For this review, take the finished solid that the model builds, in its own axes (mm). A direction names the side the tool comes from. Round coordinates to 2 decimals unless told otherwise and drop trailing zeros. Order: outer loops, then holes, each group sorted by start corner. A loop starts at its lowest first (then second) coordinate and runs counter-clockwise, first axis right, second up. Notation, with made-up numbers: (45, 49.5) - (53, 49.5) arc R14 ccw to (53, 73.5) - close; hole circle Ø9 at (29, 42). An arc over 180 degrees is marked (long way). One line per item, written item: value.
Autodesk Inventor part; units mm, degrees
ref_plane "YZ Plane" through (0, 0, 0) normal (1, 0, 0) x (0, 1, 0)
ref_plane "XZ Plane" through (0, 0, 0) normal (0, 1, 0) x (-1, 0, 0)
ref_plane "XY Plane" through (0, 0, 0) normal (0, 0, 1) x (1, 0, 0)
sketch "Эскиз1" plane through (0, 0, 0) normal (0, 0, 1) x (1, 0, 0)
  line L0 (1380.315, -1246.7097) -> (1380.315, -1245.7097)
  line L1 (1390.315, -1235.7097) -> (1440.315, -1235.7097)
  line L2 (1450.315, -1245.7097) -> (1450.315, -1246.7097)
  arc A0 (1390.315, -1235.7097) -> (1380.315, -1245.7097) centre (1390.315, -1245.7097) ccw
  arc A1 (1450.315, -1245.7097) -> (1440.315, -1235.7097) centre (1440.315, -1245.7097) ccw
  line L3 (1380.315, -1246.7097) -> (1380.315, -1247.7097)
  line L4 (1372.315, -1255.7097) -> (1357.315, -1255.7097)
  line L5 (1473.3109, -1255.7097) -> (1458.315, -1255.7097)
  line L6 (1450.315, -1247.7097) -> (1450.315, -1246.7097)
  arc A2 (1372.315, -1255.7097) -> (1380.315, -1247.7097) centre (1372.315, -1247.7097) ccw
  arc A3 (1450.315, -1247.7097) -> (1458.315, -1255.7097) centre (1458.315, -1247.7097) ccw
  circle A4 centre (1415.315, -1239.7097) radius 2
  line L7 (1357.315, -1255.7097) -> (1356.315, -1255.7097)
  arc A5 (1356.315, -1255.7097) -> (1354.315, -1257.7097) centre (1356.315, -1257.7097) ccw
  line L8 (1473.3109, -1255.7097) -> (1474.3062, -1255.7097)
  arc A6 (1476.3062, -1257.7097) -> (1474.3062, -1255.7097) centre (1474.3062, -1257.7097) ccw
  circle A7 centre (1427.315, -1239.7097) radius 2
  arc A8 (1366.3109, -1262.2097) -> (1366.3109, -1266.2097) centre (1366.3109, -1264.2097) ccw
  arc A9 (1464.3109, -1266.2097) -> (1464.3109, -1262.2097) centre (1464.3109, -1264.2097) ccw
  line L9 (1366.3109, -1262.2097) -> (1464.3109, -1262.2097)
  line L10 (1464.3109, -1266.2097) -> (1366.3109, -1266.2097)
  line L11 (1366.315, -1269.7097) -> (1464.3062, -1269.7097)
  line L12 (1476.3062, -1257.7097) -> (1476.3062, -1257.7097)
  line L13 (1354.315, -1257.7097) -> (1354.315, -1257.7097)
  arc A10 (1354.315, -1257.7097) -> (1366.315, -1269.7097) centre (1366.315, -1257.7097) ccw
  arc A11 (1464.3062, -1269.7097) -> (1476.3062, -1257.7097) centre (1464.3062, -1257.7097) ccw
  circle A12 centre (1403.315, -1239.7097) radius 2
  point P0 (0, 0)
  point P1 (1450.315, -1235.7097)
  point P2 (1380.315, -1255.7097)
  point P3 (1354.315, -1255.7097)
  point P4 (1476.3109, -1270.2097)
extrude "Выдавливание3" add sketch "Эскиз1" along normal blind 2
properties part number "NEW Бампер"
Item 1: Take a section at C-C (z = 1.65). Write out the cut boundary in (x, y) (3 decimals), plus the area to 3 significant figures.
Returned:
outline: (1354.315, -1257.71) arc R12 ccw to (1366.315, -1269.71) - (1464.306, -1269.71) arc R12 ccw to (1476.306, -1257.71) arc R2 ccw to (1474.306, -1255.71) - (1458.315, -1255.71) arc R8 cw to (1450.315, -1247.71) - (1450.315, -1245.71) arc R10 ccw to (1440.315, -1235.71) - (1390.315, -1235.71) arc R10 ccw to (1380.315, -1245.71) - (1380.315, -1247.71) arc R8 cw to (1372.315, -1255.71) - (1356.315, -1255.71) arc R2 ccw to start; hole (1366.311, -1266.21) - (1464.311, -1266.21) arc R2 ccw to (1464.311, -1262.21) - (1366.311, -1262.21) arc R2 ccw to start; hole circle Ø4 at (1403.315, -1239.71); hole circle Ø4 at (1415.315, -1239.71); hole circle Ø4 at (1427.315, -1239.71)
area: 2,590 mm^2
Item 2: Wall thickness on line 1 (Y direction, x = 1418.5, z = 1.9); line 2 (Y direction, x = 1402.5, z = 0.5); line 3 (X direction, y = -1265, z = 0.2): over which ranges is each line inside the solid? List them lowest first.
Returned:
line 1: -1269.71 to -1266.21, -1262.21 to -1235.71
line 2: -1269.71 to -1266.21, -1262.21 to -1241.54, -1237.88 to -1235.71
line 3: 1356.78 to 1364.47, 1466.15 to 1473.84
Item 3: For P1, Ø0.6, axis at y = -1246.5, z = 1.5, coming from the +X side (3 decimals); P2, Ø0.6, axis at y = -1246.5, z = 1, coming from the -X side (3 decimals); P3, Ø1, axis at x = 1362.5, z = 0.5, coming from the +Y side, all flat-tipped, find the tip position at first contact; note any pin that passes through.
Returned:
P1: x = 1450.315
P2: x = 1380.315
P3: y = -1255.71
Item 4: Machinability: for faces 4 (the flat face through (1416, -1266.21, 1)), 5 (the flat face through (1450.315, -1247, 1)), 6 (the cylindrical face through (1357.924, -1266.288, 0.986)), 7 (the flat face through (1364, -1255.71, 1)), which of the approach directions +Z, -Z, +X, -X, +Y, -Y give a long, thin tool a straight path to every point of the face, cutting with its end or side? Answer none if there is none.
Returned:
face 4: +Z, -Z
face 5: +Z, -Z, +X, +Y
face 6: +Z, -Z, -X, -Y
face 7: +Z, -Z, -X, +Y
Item 5: The part is to be moulded in two halves that separate along Y. For faces 1 (the cylindrical face through (1452.72, -1253.43, 0.99)), 2 (the flat face through (1415, -1262.21, 1)), 3 (the flat face through (1414, -1252, 0)), say which applies: +Y half, -Y half, draft (parallel to the pull), parting line (faces both ways), or undercut.
Returned:
face 1: +Y half
face 2: undercut
face 3: draft
Item 6: Take a section at B-B (y = -1264). Write out the cut boundary in (x, z).
Returned:
outline: (1356.1, 0) - (1364.32, 0) - (1364.32, 2) - (1356.1, 2) - close; (1466.3, 0) - (1474.53, 0) - (1474.53, 2) - (1466.3, 2) - close
Item 7: Take a section at D-D (y = -1253). Write out the cut boundary in (x, z), plus the area to 3 significant figures.
Returned:
outline: (1378.32, 0) - (1452.31, 0) - (1452.31, 2) - (1378.32, 2) - close
area: 148 mm^2
Item 8: Take a section at A-A (x = 1419). Write out the cut boundary in (y, z).
Returned:
outline: (-1269.71, 0) - (-1266.21, 0) - (-1266.21, 2) - (-1269.71, 2) - close; (-1262.21, 0) - (-1235.71, 0) - (-1235.71, 2) - (-1262.21, 2) - close
